from build123d import *

# Parameters (mm, degrees)
BOSS_EXTRUDE1_DEPTH = 12.7
SKETCH2_W           = 637.164894533
SKETCH2_H           = 6.35
CUT_EXTRUDE1_DEPTH  = 6.35


with BuildPart() as part:
    # Sketch1 → Boss-Extrude1 (new body)
    with BuildSketch(Plane.XY):
        Polygon((609.6, 88.9), (596.9, 88.9), (596.9, 76.2), (609.6, 76.2), (609.6, 63.5), (596.9, 63.5), (596.9, 50.8), (609.6, 50.8), (609.6, 38.1), (596.9, 38.1), (596.9, 25.4), (609.6, 25.4), (609.6, 12.7), (596.9, 12.7), (596.9, 0), (12.7, 0), (12.7, 12.7), (0, 12.7), (0, 25.4), (12.7, 25.4), (12.7, 38.1), (0, 38.1), (0, 50.8), (12.7, 50.8), (12.7, 63.5), (0, 63.5), (0, 76.2), (12.7, 76.2), (12.7, 88.9), (0, 88.9), (0, 101.6), (609.6, 101.6), align=None)
    extrude(amount=BOSS_EXTRUDE1_DEPTH)

    # Sketch2 → Cut-Extrude1 (cut)
    with BuildSketch(Plane.XY):
        with Locations((307.699845939, 15.875)):
            Rectangle(SKETCH2_W, SKETCH2_H)
    extrude(amount=CUT_EXTRUDE1_DEPTH, mode=Mode.SUBTRACT)


solid = part.part
The listing builds one solid part. Answer for the finished solid, in the listing's coordinates (mm). A direction names the side the tool comes from. Give positions to 0.01 mm unless a question says otherwise; leave off trailing zeros. Write each loop counter-clockwise with the first axis right and the second up, starting at its lowest first coordinate (ties: lowest second). Pieces come first, ordered by that corner, then holes. Notation, with made-up numbers: (-40, -23.75) - (4, -23.75) arc R30 cw to (4, 10.25) - close; hole circle Ø10 at (-3, 51). An arc over 180 degrees is marked (long way). Use a Markdown table: item, result.
1. For a pull along Y with two mould halves and no side action, classify faces 1 (the flat face through (596.9, 83, 6)), 2 (the flat face through (0, 95, 6)), 3 (the flat face through (301, 101.6, 6)) as released by +Y, released by -Y, zero draft, split by the parting line, or undercut.
Values follow:
| item | result |
|---|---|
| face 1 | undercut |
| face 2 | zero draft |
| face 3 | released by +Y |
2. Each of these flat-tipped pins is pushed along its axis until it touches: P1, Ø6.5, axis at y = 57, z = 5.5, coming from the -X side; P2, Ø5, axis at x = 9, z = 8, coming from the -Y side; P3, Ø6.5, axis at y = 56, z = 7.5, coming from the +X side. Where does it stop, or does it pass through?
Values follow:
| item | result |
|---|---|
| P1 | stops at x = 12.7 |
| P2 | stops at y = 12.7 |
| P3 | stops at x = 596.9 |
3. A tool of negligible diameter and unlimited length cuts with its end or side. For faces 4 (the flat face through (6, 88.9, 6)), 5 (the flat face through (609.6, 70, 6)), 6 (the flat face through (0, 70, 6)), 7 (the flat face through (603, 63.5, 6)), 8 (the flat face through (12.7, 6, 6)), from which of +Z, -Z, +X, -X, +Y, -Y can it reach the whole face along a straight path? Write none if from no direction.
Values follow:
| item | result |
|---|---|
| face 4 | +Z, -Z, -X |
| face 5 | +Z, -Z, +X, +Y, -Y |
| face 6 | +Z, -Z, -X, +Y, -Y |
| face 7 | +Z, -Z, +X |
| face 8 | +Z, -Z, -X, -Y |
4. Section B-B on x = 76 is taken. Write down the section's boundary in (y, z), plus the area to 3 significant figures.
Values follow:
| item | result |
|---|---|
| outline | (0, 0) - (12.7, 0) - (12.7, 6.35) - (19.05, 6.35) - (19.05, 0) - (101.6, 0) - (101.6, 12.7) - (0, 12.7) - close |
| area | 1,250 mm² |
5. Section C-C on y = 56.5 is taken. Write down the section's boundary in (x, z).
Values follow:
| item | result |
|---|---|
| outline | (12.7, 0) - (596.9, 0) - (596.9, 12.7) - (12.7, 12.7) - close |
6. Find the intervals of material crossed by probe 1 along Y at (x, z) = (219.5, 3); probe 2 along X at (y, z) = (32.5, 1), in increasing order. Write a range as from..to.
Values follow:
| item | result |
|---|---|
| probe 1 | y = 0..12.7, 19.05..101.6 |
| probe 2 | x = 12.7..596.9 |
